```python
from build123d import *

# Parameters (mm, degrees)
RESSALTO_EXTRUS_O1_DEPTH = 15
ESBO_O2_R                = 2
CORTE_EXTRUS_O1_DEPTH    = 15
ESBO_O3_R                = 2
CORTE_EXTRUS_O2_DEPTH    = 10


with BuildPart() as part:
    # Esboço1 → Ressalto-extrusão1 (new body)
    with BuildSketch(Plane.XY):
        Polygon((0, 0), (25, 0), (25, -1), (-1, -1), (-1, 25), (0, 25), align=None)
    extrude(amount=RESSALTO_EXTRUS_O1_DEPTH)

    # Esboço2 → Corte-extrusão1 (cut)
    with BuildSketch(Plane(origin=(0, 0, 0), x_dir=(0, 0, -1), z_dir=(1, 0, 0))):
        with Locations((-7.5, 12)):
            Circle(ESBO_O2_R)
    extrude(amount=-CORTE_EXTRUS_O1_DEPTH, mode=Mode.SUBTRACT)

    # Esboço3 → Corte-extrusão2 (cut)
    with BuildSketch(Plane(origin=(0, 0, 0), x_dir=(1, 0, 0), z_dir=(0, 1, 0))):
        with Locations((10, -7.5)):
            Circle(ESBO_O3_R)
    extrude(amount=-CORTE_EXTRUS_O2_DEPTH, mode=Mode.SUBTRACT)


solid = part.part
```
Could you check a few things on this model? Use its own coordinates, in mm. A direction names the side the tool comes from. Coordinates: 2 decimals unless noted, no trailing zeros. Order: outer loops, then holes, each group sorted by start corner. A loop starts at its lowest first (then second) coordinate and runs counter-clockwise, first axis right, second up. Notation, with made-up numbers: M 18,8 L 32,8 A19 cw 32,22 Z; hole C 46.5,76.25 d10. An arc over 180 degrees is marked long. Use one line per item in the form item = value. Start each with the question number.
1. Please list where these lines run through material, in increasing order: line 1 (Y direction, x = -0.4, z = 7.5); line 2 (Z direction, x = 10, y = -0.45); line 3 (X direction, y = 11.25, z = 1).
2. Suppose I cut it at B-B on z = 7.5. Write out the boundary of the cut face in (x, y), then the cut area to 3 significant figures.
3. Suppose I cut it at D-D on z = 11.5. Write out the boundary of the cut face in (x, y), then the cut area to 3 significant figures.
4. For pin 1 (4.5 mm diameter, centred on x = 10, z = 7.5, fed in from +Y); pin 2 (1 mm diameter, centred on y = 14.5, z = 9, fed in from +X), each with a flat end and sliding along its axis, tell me the tip position at first contact or that it passes through.
5. On a 3-axis mill with a long thin cutter (end or side, diameter ignored), from which of +Z, -Z, +X, -X, +Y, -Y can I reach the whole of each face in a straight line? I mean faces 1 (the flat face through (-1, 15, 7)), 2 (the flat face through (12.3, 0, 7.4)). Say none if no direction works.
6. We'd pull the mould along Z, two halves only. Please class faces 3 (the flat face through (-0.5, 25, 7.4)), 4 (the flat face through (6.3, -0.5, 15)), 5 (the cylindrical face through (9.74, -0.493, 5.517)), 6 (the flat face through (6.3, -0.5, 0)): +Z half, -Z half, draft (parallel to the pull), parting line (faces both ways), or undercut.
7. Suppose I cut it at A-A on y = 12. Write out the boundary of the cut face in (x, z), then the cut area to 3 significant figures.
Geometry says:
q1.line_1 = -1 to 10, 14 to 25
q1.line_2 = 0 to 5.5, 9.5 to 15
q1.line_3 = -1 to 0
q2.outline = M -1,-1 L 8,-1 L 8,0 L 0,0 L 0,10 L -1,10 Z; M -1,14 L 0,14 L 0,25 L -1,25 Z; M 12,-1 L 25,-1 L 25,0 L 12,0 Z
q2.area = 43.0 mm^2
q3.outline = M -1,-1 L 25,-1 L 25,0 L 0,0 L 0,25 L -1,25 Z
q3.area = 51.0 mm^2
q4.pin_1 = 0
q4.pin_2 = 0
q5.face_1 = +Z, -Z, -X, +Y, -Y
q5.face_2 = +Z, -Z, +X, +Y
q6.face_3 = draft
q6.face_4 = +Z half
q6.face_5 = undercut
q6.face_6 = -Z half
q7.outline = M -1,0 L 0,0 L 0,5.5 L -1,5.5 Z; M -1,9.5 L 0,9.5 L 0,15 L -1,15 Z
q7.area = 11.0 mm^2
